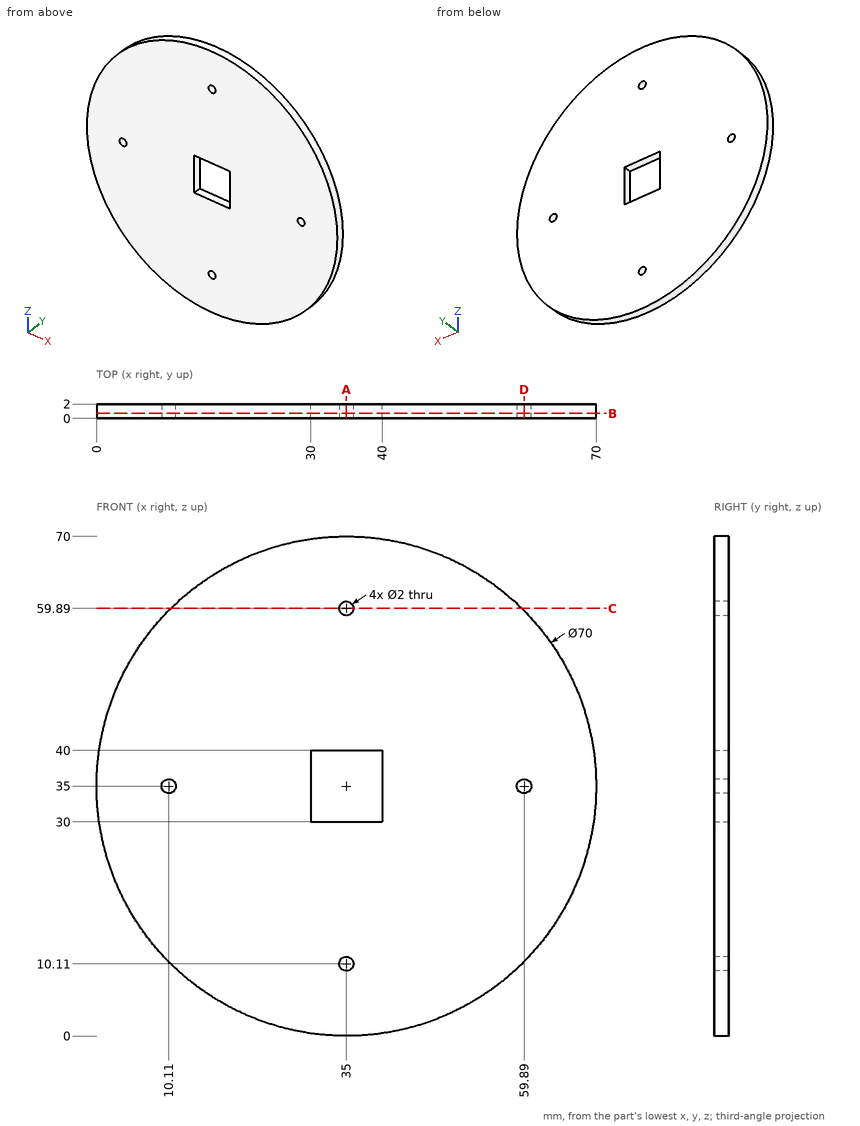
Verification items for this drawing (mm, ordinates from the low corner). Give positions to 0.01 mm unless a question says otherwise; leave off trailing zeros. Write each loop counter-clockwise with the first axis right and the second up, starting at its lowest first coordinate (ties: lowest second). Pieces come first, ordered by that corner, then holes.
1) Section check B-B, the plane y = 0.7. Record the boundary of the cut face in (x, z), and give its area (3 significant figures).
2) Section check D-D, the plane x = 59.89. Record the boundary of the cut face in (y, z).
3) Material ranges on L1, parallel to Z at x = 35, y = 0.95; L2, parallel to Z at x = 10.11, y = 0.8, recorded low to high.
4) Gauge pin test, flat ends, axial feed: pin 1 (1.6 mm diameter, centred on x = 10.11, z = 35, fed in from +Y); pin 2 (0.6 mm diameter, centred on x = 33.5, y = 1, fed in from -Z). Record the tip position at first contact, or that the pin passes through.
5) Section check C-C, the plane z = 59.89. Record the boundary of the cut face in (x, y), and give its area (3 significant figures).
6) Section check A-A, the plane x = 35. Record the boundary of the cut face in (y, z), and give its area (3 significant figures).
Computed:
1. outline: circle Ø70 at (35, 35); hole circle Ø2 at (10.11, 35); hole (30, 30) - (40, 30) - (40, 40) - (30, 40) - close; hole circle Ø2 at (35, 10.11); hole circle Ø2 at (35, 59.89); hole circle Ø2 at (59.89, 35)
1. area: 3,740 mm2
2. outline: (0, 10.39) - (2, 10.39) - (2, 34) - (0, 34) - close; (0, 36) - (2, 36) - (2, 59.61) - (0, 59.61) - close
3. L1: z = 0 to 9.11, 11.11 to 30, 40 to 58.89, 60.89 to 70
3. L2: z = 10.39 to 34, 36 to 59.61
4. pin 1: passes through
4. pin 2: stops at z = 0.02
5. outline: (10.39, 0) - (34, 0) - (34, 2) - (10.39, 2) - close; (36, 0) - (59.61, 0) - (59.61, 2) - (36, 2) - close
5. area: 94.4 mm2
6. outline: (0, 0) - (2, 0) - (2, 9.11) - (0, 9.11) - close; (0, 11.11) - (2, 11.11) - (2, 30) - (0, 30) - close; (0, 40) - (2, 40) - (2, 58.89) - (0, 58.89) - close; (0, 60.89) - (2, 60.89) - (2, 70) - (0, 70) - close
6. area: 112 mm2
